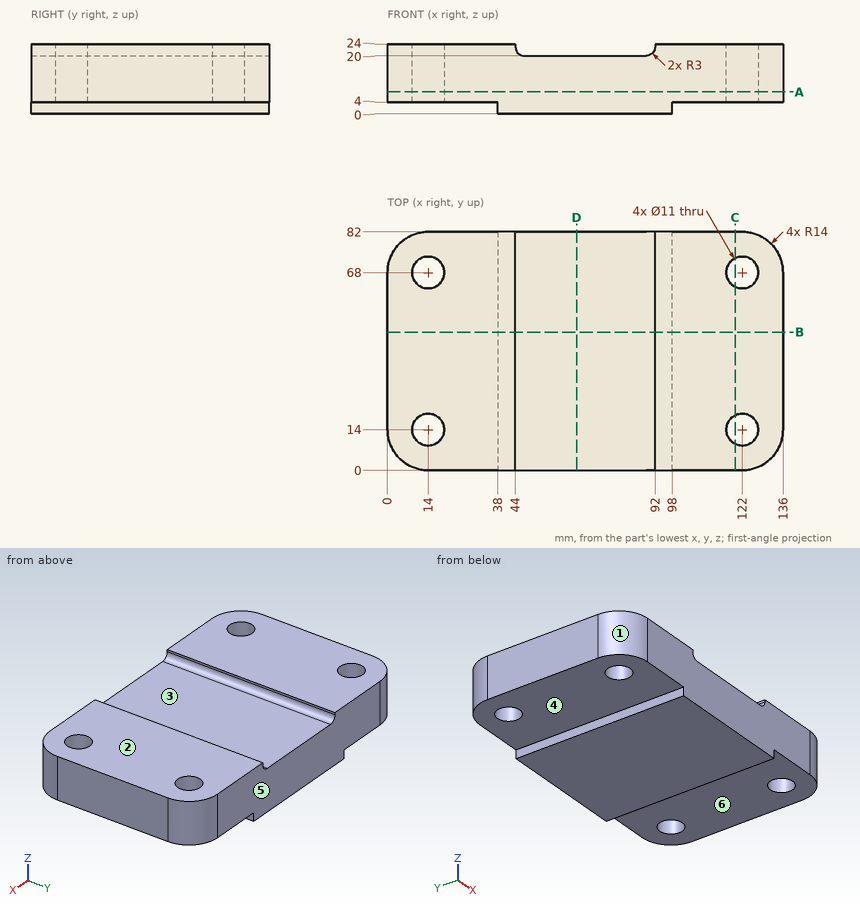
Input: dimensioned drawing with shaded views. Units: mm. Origin: part minimum x, y, z. A direction names the side the tool comes from. Give positions to 0.01 mm unless a question says otherwise; leave off trailing zeros. Order: outer loops, then holes, each group sorted by start corner. A loop starts at its lowest first (then second) coordinate and runs counter-clockwise, first axis right, second up. Notation, with made-up numbers: (-1, 11.25) -> (10, 11.25) arc R25 ccw to (10, 46.25) -> close; hole circle Ø11 at (24.25, -11). An arc over 180 degrees is marked (long way). Use one line per item in the form item = value.
1) Section C-C, the plane x = 119.5. Return loops of the section in (y, z).
Response values:
outline = (0, 4) -> (9.1, 4) -> (9.1, 24) -> (0, 24) -> close; (18.9, 4) -> (63.1, 4) -> (63.1, 24) -> (18.9, 24) -> close; (72.9, 4) -> (82, 4) -> (82, 24) -> (72.9, 24) -> close
2) Mould query, pull axis X, two halves, no side actions, for the marked faces 1, 2 and 3. Classes: pulls with the +X half, pulls with the -X half, needs draft (parallel to the pull), parting line crosses it, or undercut.
Response values:
face_1 = pulls with the -X half
face_2 = needs draft
face_3 = undercut
3) Reachability of the marked faces 4, 5 and 6 from +Z, -Z, +X, -X, +Y, -Y: full face, straight path, thin tool, end or side. Return the list, or none.
Response values:
face_4 = -Z, -X, +Y, -Y
face_5 = +Z, -Z, +X, -X, +Y
face_6 = -Z, +X, +Y, -Y
4) Section A-A, the plane z = 7.5. Return loops of the section in (x, y), and give its area (3 significant figures).
Response values:
outline = (0, 14) arc R14 ccw to (14, 0) -> (122, 0) arc R14 ccw to (136, 14) -> (136, 68) arc R14 ccw to (122, 82) -> (14, 82) arc R14 ccw to (0, 68) -> close; hole circle Ø11 at (14, 14); hole circle Ø11 at (14, 68); hole circle Ø11 at (122, 14); hole circle Ø11 at (122, 68)
area = 10,600 mm^2
5) First-contact query: pin 1 Ø12 at (x, y) = (122, 69) entering from +Z; pin 2 Ø1.2 at (y, z) = (25.5, 2) entering from -X; pin 3 Ø3 at (y, z) = (29, 2) entering from +X; pin 4 Ø1.5 at (x, y) = (121.5, 56) entering from -Z. Flat tips, straight axial feed; report the tip coordinate or a pass-through.
Response values:
pin_1 = 24
pin_2 = 38
pin_3 = 98
pin_4 = 4
6) Line query: probe 1 along Y at (x, z) = (122, 17.5); probe 2 along X at (y, z) = (68, 8.5); probe 3 along Y at (x, z) = (117, 14.75). Output: solid intervals per line, ascending.
Response values:
probe_1 = 0 to 8.5, 19.5 to 62.5, 73.5 to 82
probe_2 = 0 to 8.5, 19.5 to 116.5, 127.5 to 136
probe_3 = 0 to 11.71, 16.29 to 65.71, 70.29 to 82
7) Section D-D, the plane x = 65. Return loops of the section in (y, z).
Response values:
outline = (0, 0) -> (82, 0) -> (82, 20) -> (0, 20) -> close
8) Section B-B, the plane y = 47.5. Return loops of the section in (x, z), and give its area (3 significant figures).
Response values:
outline = (0, 4) -> (38, 4) -> (38, 0) -> (98, 0) -> (98, 4) -> (136, 4) -> (136, 24) -> (92, 24) -> (92, 23) arc R3 cw to (89, 20) -> (47, 20) arc R3 cw to (44, 23) -> (44, 24) -> (0, 24) -> close
area = 2,770 mm^2
